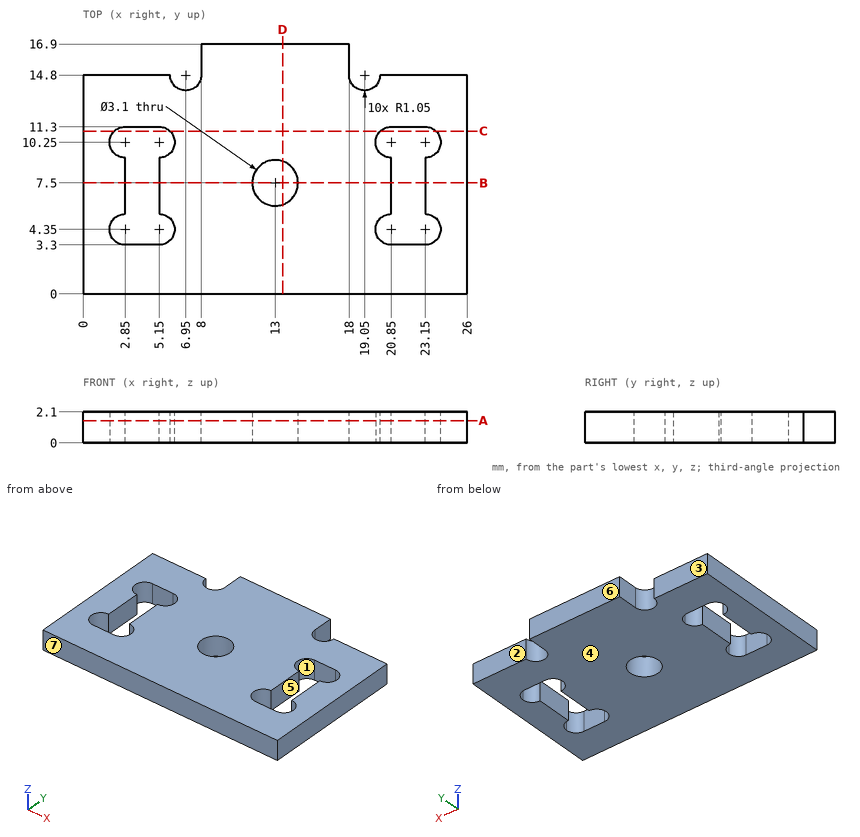
Job drawing, mm, ordinate dimensions from the low corner. One solid piece. A direction names the side the tool comes from. Coordinates: 2 decimals unless noted, no trailing zeros. Loops run counter-clockwise (first coordinate to the right, second up) from the corner with the lowest first, then second, coordinate; pieces in that order, holes last. Notation, with made-up numbers: (-1.75, 62.5) - (48.25, 62.5) arc R21 ccw to (48.25, 86.5) - close; hole circle Ø1 at (76, 2). An arc over 180 degrees is marked (long way). Write item = value, one per line. Start each with the question number.
Q1. Which spindle directions (+Z, -Z, +X, -X, +Y, -Y) get a long thin tool onto all of the face, cutting with end or side? Do the marked faces 1, 2 and 3. Say none if no direction does.
Q2. Cut at C-C, the plane y = 11. List the corners of the cut face in (x, z), then the cut area to 3 significant figures.
Q3. Cut at B-B, the plane y = 7.5. List the corners of the cut face in (x, z).
Q4. Cut at D-D, the plane x = 13.5. List the corners of the cut face in (y, z).
Q5. Cut at A-A, the plane z = 1.5. List the corners of the cut face in (x, y).
Q6. Pull direction Y, two halves, no side cores. Call the marked faces 4, 5, 6 and 7: pulls with the +Y half, pulls with the -Y half, needs draft (parallel to the pull), parting line crosses it, or undercut.
Q7. Flat gauge pins, fed straight in: pin 1 Ø1 at (y, z) = (15.5, 1.5) entering from -X; pin 2 Ø1 at (x, z) = (22, 1.5) entering from +Y. Where does each tip first touch, or does it go through?
Q8. Drill centre lines: L1, parallel to X at y = 5.75, z = 0.45; L2, parallel to Y at x = 3, z = 0.75; L3, parallel to Y at x = 13, z = 0.75. Where is each one in solid material? Low to high.
Computed:
q1.face_1 = +Z, -Z
q1.face_2 = +Z, -Z, +X, +Y
q1.face_3 = +Z, -Z, -X, +Y
q2.outline = (0, 0) - (2.12, 0) - (2.12, 2.1) - (0, 2.1) - close; (5.88, 0) - (20.12, 0) - (20.12, 2.1) - (5.88, 2.1) - close; (23.88, 0) - (26, 0) - (26, 2.1) - (23.88, 2.1) - close
q2.area = 38.8 mm²
q3.outline = (0, 0) - (2.85, 0) - (2.85, 2.1) - (0, 2.1) - close; (5.15, 0) - (11.45, 0) - (11.45, 2.1) - (5.15, 2.1) - close; (14.55, 0) - (20.85, 0) - (20.85, 2.1) - (14.55, 2.1) - close; (23.15, 0) - (26, 0) - (26, 2.1) - (23.15, 2.1) - close
q4.outline = (0, 0) - (6.03, 0) - (6.03, 2.1) - (0, 2.1) - close; (8.97, 0) - (16.9, 0) - (16.9, 2.1) - (8.97, 2.1) - close
q5.outline = (0, 0) - (26, 0) - (26, 14.8) - (20.1, 14.8) arc R1.05 cw to (18, 14.8) - (18, 16.9) - (8, 16.9) - (8, 14.8) arc R1.05 cw to (5.9, 14.8) - (0, 14.8) - close; hole (2.85, 3.3) - (5.15, 3.3) arc R1.05 ccw to (5.15, 5.4) - (5.15, 9.2) arc R1.05 ccw to (5.15, 11.3) - (2.85, 11.3) arc R1.05 ccw to (2.85, 9.2) - (2.85, 5.4) arc R1.05 ccw to start; hole circle Ø3.1 at (13, 7.5); hole (20.85, 3.3) - (23.15, 3.3) arc R1.05 ccw to (23.15, 5.4) - (23.15, 9.2) arc R1.05 ccw to (23.15, 11.3) - (20.85, 11.3) arc R1.05 ccw to (20.85, 9.2) - (20.85, 5.4) arc R1.05 ccw to start
q6.face_4 = needs draft
q6.face_5 = undercut
q6.face_6 = pulls with the +Y half
q6.face_7 = pulls with the -Y half
q7.pin_1 = 8
q7.pin_2 = 14.8
q8.L1 = 0 to 2.85, 5.15 to 20.85, 23.15 to 26
q8.L2 = 0 to 3.3, 11.3 to 14.8
q8.L3 = 0 to 5.95, 9.05 to 16.9
